```python
from build123d import *

# Parameters (mm, degrees)
BOSS_EXTRUDE1_DEPTH     = 1.6
SKETCH2_W               = 2.54
SKETCH2_H               = 1.27
BOSS_EXTRUDE2_DEPTH     = 0.1
SKETCH3_W               = 14.62
SKETCH3_H               = 6.07
BOSS_EXTRUDE3_DEPTH     = 5
SKETCH4_R               = 2.49
SKETCH4_R_2             = 1.795
BOSS_EXTRUDE5_DEPTH     = 2.52
CUT_EXTRUDE1_DEPTH      = 17.929090348
CUT_EXTRUDE1_DEPTH_BACK = 17.929090348
SKETCH5_R               = 1.25


with BuildPart() as part:
    # Sketch1 → Boss-Extrude1 (new body)
    with BuildSketch(Plane(origin=(0, 0, 0), x_dir=(1, 0, 0), z_dir=(0, 1, 0))):
        with BuildLine():
            Line((12, 5.5), (-12, 5.5))
            ThreePointArc((-12, 5.5), (-12.707106781, 5.207106781), (-13, 4.5))
            Line((-13, 4.5), (-13, -4.5))
            ThreePointArc((-13, -4.5), (-12.707106781, -5.207106781), (-12, -5.5))
            Line((-12, -5.5), (12, -5.5))
            ThreePointArc((12, -5.5), (12.707106781, -5.207106781), (13, -4.5))
            Line((13, -4.5), (13, 4.5))
            ThreePointArc((13, 4.5), (12.707106781, 5.207106781), (12, 5.5))
        make_face()
    extrude(amount=BOSS_EXTRUDE1_DEPTH)

    # Sketch2 → Boss-Extrude2 (add)
    with BuildSketch(Plane(origin=(0, 1.6, 0), x_dir=(1, 0, 0), z_dir=(0, 1, 0))):
        with Locations((10.34, 4.08)):
            Rectangle(SKETCH2_W, SKETCH2_H)
        with Locations((10.34, -2.61)):
            Rectangle(SKETCH2_W, SKETCH2_H)
    extrude(amount=BOSS_EXTRUDE2_DEPTH)

    # Sketch3 → Boss-Extrude3 (add)
    with BuildSketch(Plane(origin=(0, 1.6, 0), x_dir=(1, 0, 0), z_dir=(0, 1, 0))):
        with Locations((-5.38, 2.12)):
            Rectangle(SKETCH3_W, SKETCH3_H)
    extrude(amount=BOSS_EXTRUDE3_DEPTH)

    # Sketch4 → Boss-Extrude5 (add)
    with BuildSketch(Plane.ZY.offset(12.69)):
        with Locations(Location((-2.12, 4.1, 0), (0, 0, 180))):
            Circle(SKETCH4_R)
        with Locations((-2.12, 4.1)):
            Circle(SKETCH4_R_2, mode=Mode.SUBTRACT)
    extrude(amount=BOSS_EXTRUDE5_DEPTH)

    # Sketch5 → Cut-Extrude1 (cut, two sides: drawn at the far end of the back side and taken through both)
    with BuildSketch(Plane(origin=(0, 1.6, 0), x_dir=(1, 0, 0), z_dir=(0, 1, 0)).offset(-CUT_EXTRUDE1_DEPTH_BACK)):
        with Locations(Location((5.5, -0.75, 0), (0, 0, 270))):
            Circle(SKETCH5_R)
    extrude(amount=CUT_EXTRUDE1_DEPTH + CUT_EXTRUDE1_DEPTH_BACK, mode=Mode.SUBTRACT)


solid = part.part
```
Could you check a few things on this model? Use its own coordinates, in mm. A direction names the side the tool comes from. Round coordinates to 2 decimals unless told otherwise and drop trailing zeros. Loops run counter-clockwise (first coordinate to the right, second up) from the corner with the lowest first, then second, coordinate; pieces in that order, holes last.
Q1. Please list where these lines run through material, in increasing order: L1, parallel to Z at x = 5.5, y = 0.5; L2, parallel to Y at x = -13.85, z = -2.12 (3 decimals); L3, parallel to X at y = 1.75, z = -2.5.
Q2. Thinking about a two-plate mould opening in X: for faces 1 (the flat face through (13, 1, 0)), 2 (the flat face through (-13, 1, 0)), 3 (the flat face through (0, 0, 0)), 4 (the cylindrical face through (4.28, 0.79, 0.48)), which applies, pulls with the +X half, pulls with the -X half, needs draft (parallel to the pull), parting line crosses it, or undercut?
Q3. For P1, Ø1.5, axis at x = -9.5, y = 4.5, coming from the +Z side (3 decimals); P2, Ø1, axis at y = 2, z = -2, coming from the +X side; P3, Ø1, axis at x = 10, z = -4.5, coming from the +Y side; P4, Ø3, axis at x = -11, y = 4.5, coming from the -Z side (3 decimals), each with a flat end and sliding along its axis, tell me the tip position at first contact or that it passes through.
Q4. I want a section at A-A (x = 5.5). Write out the boundary of the cut face in (y, z).
Q5. I want a section at B-B (z = -2.12). Write out the boundary of the cut face in (x, y) (3 decimals).
Q6. I want a section at C-C (x = -0.25). Write out the boundary of the cut face in (y, z) (3 decimals), and give its area (4 significant figures).
Q7. On a 3-axis mill with a long thin cutter (end or side, diameter ignored), from which of +Z, -Z, +X, -X, +Y, -Y can I reach the whole of each face in a straight line? I mean faces 5 (the flat face through (-5, 4, -5.155)), 6 (the cylindrical face through (12.715, 0.789, -5.199)), 7 (the flat face through (10, 1.7, -4)), 8 (the flat face through (-12.69, 4, -2)). Say none if no direction works.
Q8. I want a section at D-D (y = 4.1). Write out the boundary of the cut face in (x, z) (3 decimals).
Answer below:
1. L1: z = -5.5 to -0.5, 2 to 5.5
1. L2: y = 1.61 to 2.305, 5.895 to 6.59
1. L3: x = -15.21 to 1.93
2. face 1: pulls with the +X half
2. face 2: pulls with the -X half
2. face 3: needs draft
2. face 4: undercut
3. P1: stops at z = 0.915
3. P2: stops at x = 13
3. P3: stops at y = 1.7
3. P4: stops at z = -5.155
4. outline: (0, -5.5) - (1.6, -5.5) - (1.6, -0.5) - (0, -0.5) - close; (0, 2) - (1.6, 2) - (1.6, 5.5) - (0, 5.5) - close
5. outline: (-15.21, 1.61) - (-12.69, 1.61) - (-12.69, 1.6) - (-13, 1.6) - (-13, 0) - (13, 0) - (13, 1.6) - (1.93, 1.6) - (1.93, 6.6) - (-12.69, 6.6) - (-12.69, 6.59) - (-15.21, 6.59) - (-15.21, 5.895) - (-12.69, 5.895) - (-12.69, 2.305) - (-15.21, 2.305) - close
6. outline: (0, -5.5) - (1.6, -5.5) - (1.6, -5.155) - (6.6, -5.155) - (6.6, 0.915) - (1.6, 0.915) - (1.6, 5.5) - (0, 5.5) - close
6. area: 47.95 mm2
7. face 5: -Z, +X, -X, +Y
7. face 6: -Z, +X, +Y, -Y
7. face 7: +Z, -Z, +X, +Y
7. face 8: -X
8. outline: (-15.21, -4.61) - (-12.69, -4.61) - (-12.69, -5.155) - (1.93, -5.155) - (1.93, 0.915) - (-12.69, 0.915) - (-12.69, 0.37) - (-15.21, 0.37) - (-15.21, -0.325) - (-12.69, -0.325) - (-12.69, -3.915) - (-15.21, -3.915) - close
